The listing builds one solid part. Answer for the finished solid, in the listing's coordinates (mm). A direction names the side the tool comes from. Give positions to 0.01 mm unless a question says otherwise; leave off trailing zeros. Write each loop counter-clockwise with the first axis right and the second up, starting at its lowest first coordinate (ties: lowest second). Pieces come first, ordered by that corner, then holes. Notation, with made-up numbers: M -29,37 L -6,37 A26 ccw -6,65 Z; hole C 86,23.5 d6. An arc over 180 degrees is marked long. Return JSON: item names as keys, results as strings.
from build123d import *

# Parameters (mm, degrees)
SKETCH1_W                   = 76.2
SKETCH1_H                   = 44.45
BOSS_EXTRUDE1_DEPTH         = 4.445
SKETCH2_W                   = 76.2
SKETCH2_H                   = 1.905
BOSS_EXTRUDE2_DEPTH         = 12.7
CUT_EXTRUDE3_DEPTH          = 46.900442536
SKETCH7_W                   = 27.8765
SKETCH7_H                   = 22.225
CUT_EXTRUDE4_DEPTH          = 1.651
SKETCH11_W                  = 10.16
SKETCH11_H                  = 12.192
CUT_EXTRUDE6_DEPTH          = 3.175
SKETCH13_W                  = 76.2
SKETCH13_H                  = 17.145
BOSS_EXTRUDE3_DEPTH         = 12.7
FILLET1_R                   = 1.778
F_1_4_20_TAPPED_HOLE1_D     = 5.1054
F_1_4_20_TAPPED_HOLE1_DEPTH = 6.35
F_1_4_20_TAPPED_HOLE1_TIP   = 1.533816902
F_4_40_TAPPED_HOLE1_D       = 2.2606
F_4_40_TAPPED_HOLE1_DEPTH   = 6.35
F_4_40_TAPPED_HOLE1_TIP     = 0.679152758


with BuildPart() as part:
    # Sketch1 → Boss-Extrude1 (new body)
    with BuildSketch(Plane(origin=(0, 0, 0), x_dir=(1, 0, 0), z_dir=(0, 1, 0))):
        Rectangle(SKETCH1_W, SKETCH1_H)
    extrude(amount=BOSS_EXTRUDE1_DEPTH)

    # Sketch2 → Boss-Extrude2 (add)
    with BuildSketch(Plane(origin=(0, 4.445, 0), x_dir=(1, 0, 0), z_dir=(0, 1, 0))):
        with Locations((0, 21.2725)):
            Rectangle(SKETCH2_W, SKETCH2_H)
        with Locations((0, -21.2725)):
            Rectangle(SKETCH2_W, SKETCH2_H)
    extrude(amount=BOSS_EXTRUDE2_DEPTH)

    # Sketch6 → Cut-Extrude3 (cut, through all)
    with BuildSketch(Plane(origin=(0, 4.445, 0), x_dir=(1, 0, 0), z_dir=(0, 1, 0))):
        with BuildLine():
            Line((-8.5725, 15.6845), (-8.5725, -2.9845))
            ThreePointArc((-8.5725, -2.9845), (-8.051735857, -4.241735857), (-6.7945, -4.7625))
            Line((-6.7945, -4.7625), (6.7945, -4.7625))
            ThreePointArc((6.7945, -4.7625), (8.051735857, -4.241735857), (8.5725, -2.9845))
            Line((8.5725, -2.9845), (8.5725, 15.6845))
            ThreePointArc((8.5725, 15.6845), (8.051735857, 16.941735857), (6.7945, 17.4625))
            Line((6.7945, 17.4625), (-6.7945, 17.4625))
            ThreePointArc((-6.7945, 17.4625), (-8.051735857, 16.941735857), (-8.5725, 15.6845))
        make_face()
    extrude(amount=-CUT_EXTRUDE3_DEPTH, mode=Mode.SUBTRACT)

    # Sketch7 → Cut-Extrude4 (cut)
    with BuildSketch(Plane(origin=(0, 4.445, 0), x_dir=(1, 0, 0), z_dir=(0, 1, 0))):
        with Locations((-24.16175, 6.35)):
            Rectangle(SKETCH7_W, SKETCH7_H)
        with Locations((24.16175, 6.35)):
            Rectangle(SKETCH7_W, SKETCH7_H)
    extrude(amount=-CUT_EXTRUDE4_DEPTH, mode=Mode.SUBTRACT)

    # Sketch11 → Cut-Extrude6 (cut)
    with BuildSketch(Plane(origin=(0, 4.445, 0), x_dir=(1, 0, 0), z_dir=(0, 1, 0))):
        with Locations((-31.115, -12.7)):
            Rectangle(SKETCH11_W, SKETCH11_H)
        with Locations((31.115, -12.7)):
            Rectangle(SKETCH11_W, SKETCH11_H)
    extrude(amount=-CUT_EXTRUDE6_DEPTH, mode=Mode.SUBTRACT)

    # Sketch13 → Boss-Extrude3 (add)
    with BuildSketch(Plane.XY.offset(-20.32)):
        with Locations((0, 8.5725)):
            Rectangle(SKETCH13_W, SKETCH13_H)
    extrude(amount=-BOSS_EXTRUDE3_DEPTH)

    # Fillet1
    fillet1_edges = [part.edges().sort_by_distance(p)[0] for p in [
        (-26.035, 2.8575, 18.796),
        (-36.195, 2.8575, 18.796),
        (26.035, 2.8575, 18.796),
        (26.035, 2.8575, 6.604),
        (36.195, 2.8575, 6.604),
        (36.195, 2.8575, 18.796),
        (-10.2235, 3.6195, -17.4625),
        (-10.2235, 3.6195, 4.7625),
        (10.2235, 3.6195, -17.4625),
        (10.2235, 3.6195, 4.7625),
        (-36.195, 2.8575, 6.604),
        (-26.035, 2.8575, 6.604),
    ]]
    fillet(fillet1_edges, radius=FILLET1_R)

    # 1/4-20 Tapped Hole1
    with Locations(Plane(origin=(0, 0, -33.02), x_dir=(-1, 0, 0), z_dir=(0, 0, -1))):
        with Locations((-25.4, 8.89), (25.4, 8.89)):
            Hole(F_1_4_20_TAPPED_HOLE1_D / 2, depth=F_1_4_20_TAPPED_HOLE1_DEPTH)
            with Locations((0, 0, -(F_1_4_20_TAPPED_HOLE1_DEPTH + F_1_4_20_TAPPED_HOLE1_TIP / 2))):  # 118° drill point
                Cone(0, F_1_4_20_TAPPED_HOLE1_D / 2, F_1_4_20_TAPPED_HOLE1_TIP, mode=Mode.SUBTRACT)

    # #4-40 Tapped Hole1
    with Locations(Plane(origin=(0, 17.145, 0), x_dir=(-1, 0, 0), z_dir=(0, 1, 0))):
        with Locations((12.7, -26.67), (-12.7, -26.67)):
            Hole(F_4_40_TAPPED_HOLE1_D / 2, depth=F_4_40_TAPPED_HOLE1_DEPTH)
            with Locations((0, 0, -(F_4_40_TAPPED_HOLE1_DEPTH + F_4_40_TAPPED_HOLE1_TIP / 2))):  # 118° drill point
                Cone(0, F_4_40_TAPPED_HOLE1_D / 2, F_4_40_TAPPED_HOLE1_TIP, mode=Mode.SUBTRACT)


solid = part.part
Item 1: Which of the six approach directions +Z, -Z, +X, -X, +Y, -Y give full straight-line access (tool end or side, diameter ignored) to faces 1 (the flat face through (-26.035, 3, 13)), 2 (the flat face through (0, 2, 4.762)), 3 (the flat face through (-1, 4.445, 9)), 4 (the flat face through (24, 2.794, -7))?
Geometry results:
{"face 1": "+Y", "face 2": "+Y, -Y", "face 3": "+X, -X, +Y", "face 4": "+X, +Y"}
Item 2: Find the intervals of material crossed by line 1 (Z direction, x = 12.7, y = 13.5) (3 decimals); line 2 (X direction, y = 8.89, z = -28.5); line 3 (X direction, y = 15, z = -26.67), in increasing order.
Geometry results:
{"line 1": "z = -33.02 to -27.8, -25.54 to -20.32, 20.32 to 22.225", "line 2": "x = -38.1 to -27.95, -22.85 to 22.85, 27.95 to 38.1", "line 3": "x = -38.1 to -13.83, -11.57 to 11.57, 13.83 to 38.1"}
Item 3: Given pin 1 Ø10 at (y, z) = (4, -6) entering from +X; pin 2 Ø1 at (x, z) = (16, 5) entering from +Y (3 decimals); pin 3 Ø1.5 at (y, z) = (5.5, -16.5) entering from -X; pin 4 Ø0.5 at (y, z) = (4, -10) entering from -X, each flat-ended and moving along its own axis, determine where each tip first touches the part or whether it passes through.
Geometry results:
{"pin 1": "stops at x = 38.1", "pin 2": "stops at y = 4.445", "pin 3": "passes through", "pin 4": "stops at x = -10.22"}
Item 4: A cutting plane is placed at A-A, the plane y = 5.5. Write down the section's boundary in (x, z) (3 decimals), plus the area to 3 significant figures.
Geometry results:
{"outline": "M -38.1,-33.02 L 38.1,-33.02 L 38.1,-20.32 L -38.1,-20.32 Z; M -38.1,20.32 L 38.1,20.32 L 38.1,22.225 L -38.1,22.225 Z", "area": "1,110 mm2"}
Item 5: A cutting plane is placed at D-D, the plane z = -18.5. Write down the section's boundary in (x, y) (3 decimals).
Geometry results:
{"outline": "M -38.1,0 L 38.1,0 L 38.1,4.445 L -38.1,4.445 Z"}
Item 6: A cutting plane is placed at B-B, the plane z = 0.5. Write down the section's boundary in (x, y) (1 decimal), plus the area to 3 significant figures.
Geometry results:
{"outline": "M -38.1,0 L -8.6,0 L -8.6,4.4 L -10.2,4.4 L -10.2,2.8 L -38.1,2.8 Z; M 8.6,0 L 38.1,0 L 38.1,2.8 L 10.2,2.8 L 10.2,4.4 L 8.6,4.4 Z", "area": "170 mm2"}
Item 7: A cutting plane is placed at C-C, the plane x = -30.5. Write down the section's boundary in (y, z) (1 decimal), plus the area to 3 significant figures.
Geometry results:
{"outline": "M 0,-33 L 17.1,-33 L 17.1,-20.3 L 4.4,-20.3 L 4.4,-17.5 L 2.8,-17.5 L 2.8,4.8 L 4.4,4.8 L 4.4,6.6 L 1.3,6.6 L 1.3,18.8 L 4.4,18.8 L 4.4,20.3 L 17.1,20.3 L 17.1,22.2 L 0,22.2 Z", "area": "356 mm2"}
Item 8: Determine the mould class of faces 5 (the flat face through (-31, 3, 18.796)), 6 (the flat face through (-1, 8, 22.225)), 7 (the flat face through (-38.1, 1, -17)) for opening direction Z: +Z half, -Z half, draft (parallel to the pull), parting line (faces both ways), or undercut.
Geometry results:
{"face 5": "undercut", "face 6": "+Z half", "face 7": "draft"}
